Job drawing, mm, ordinate dimensions from the low corner. One solid piece. A direction names the side the tool comes from. Give positions to 0.01 mm unless a question says otherwise; leave off trailing zeros. One line per question, with ' | ' between items.
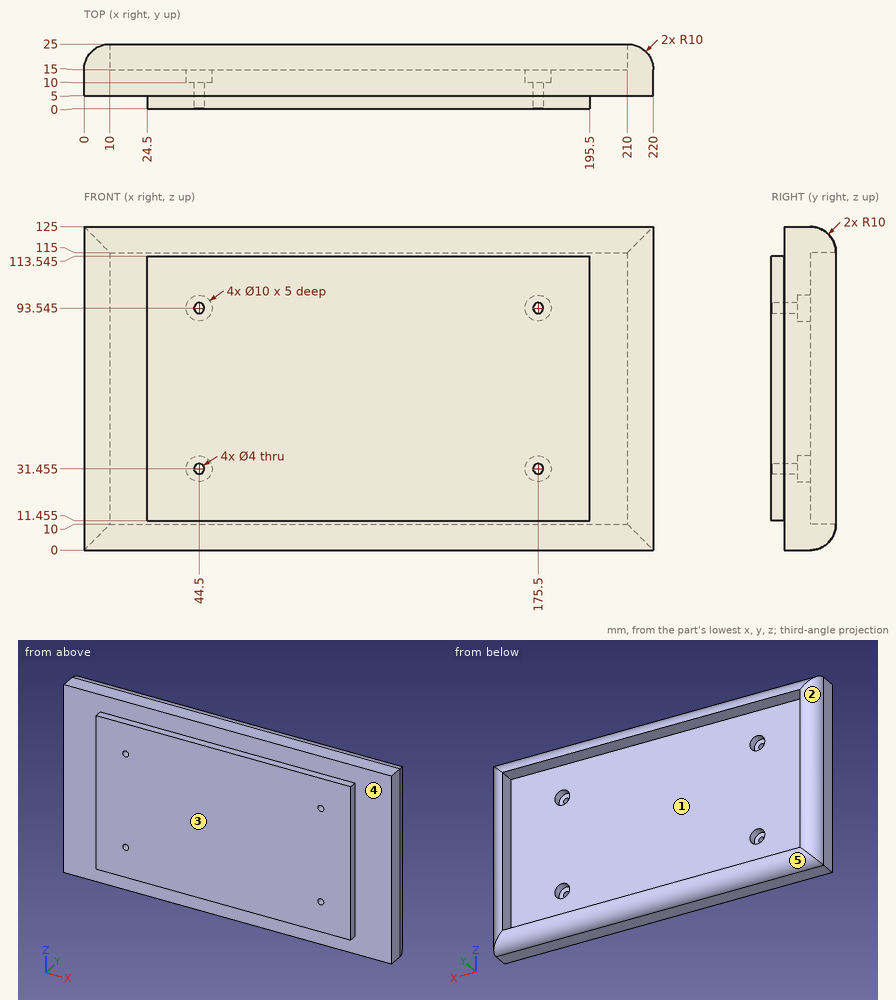
1. Tool access for the marked faces 4 and 5: list every direction of +Z, -Z, +X, -X, +Y, -Y with a clear straight run to the whole face (end or side of a thin tool).
Worked out:
face 4: -Y | face 5: -Z, +X, -X, +Y
2. Probe L1, parallel to X at y = 4, z = 89; L2, parallel to Y at x = 40.5, z = 21; L3, parallel to X at y = 23, z = 30.5. List the from-to ranges inside material, lowest first. Write a range as from..to.
Worked out:
L1: x = 24.5..195.5 | L2: y = 0..15 | L3: x = 4..10, 210..216
3. Mould opens along X. For the marked faces 1, 2 and 3 say: released by +X, released by -X, zero draft, split by the parting line, or undercut.
Worked out:
face 1: undercut | face 2: released by -X | face 3: zero draft
4. Drop flat-ended pins along their axis: pin 1 (11 mm diameter, centred on x = 176, z = 34, fed in from +Y); pin 2 (3 mm diameter, centred on y = 18.5, z = 57.5, fed in from +X); pin 3 (3 mm diameter, centred on x = 175.5, z = 91.5, fed in from +Y). Give the stop position or say it passes through.
Worked out:
pin 1: stops at y = 15 | pin 2: stops at x = 219.8 | pin 3: stops at y = 10
